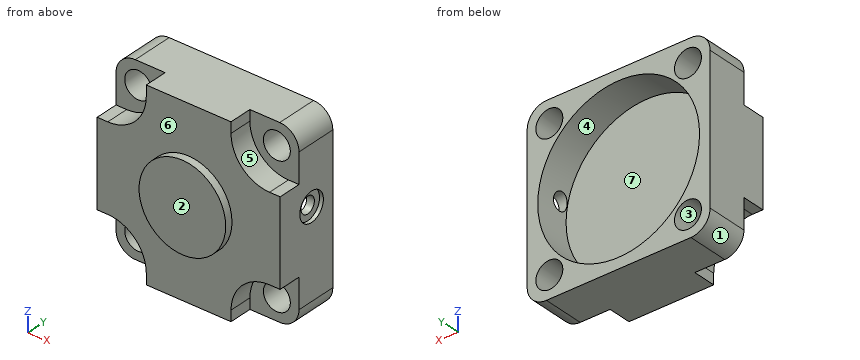
from build123d import *

# Parameters (mm, degrees)
F0_R      = 7
F1_DEPTH  = 16.75
F2_R      = 7
F3_DEPTH  = 12
F4_R      = 22.5
F5_DEPTH  = 4
F6_R      = 42
F8_DEPTH  = 18
F7_R      = 7.5
F7_R_2    = 4.25
F9_DEPTH  = 2
F10_DEPTH = 8


with BuildPart() as f1:
    # F0 (on Front) → F1 (new body, symmetric)
    with BuildSketch(Plane.XZ):
        with BuildLine():
            Line((-37.5, -47.5), (37.5, -47.5))
            ThreePointArc((37.5, -47.5), (44.5710678119, -44.5710678119), (47.5, -37.5))
            Line((47.5, -37.5), (47.5, 37.5))
            ThreePointArc((47.5, 37.5), (44.5710678119, 44.5710678119), (37.5, 47.5))
            Line((37.5, 47.5), (-37.5, 47.5))
            ThreePointArc((-37.5, 47.5), (-44.5710678119, 44.5710678119), (-47.5, 37.5))
            Line((-47.5, 37.5), (-47.5, -37.5))
            ThreePointArc((-47.5, -37.5), (-44.5710678119, -44.5710678119), (-37.5, -47.5))
        make_face()
        with Locations((-36, -36)):
            Circle(F0_R, mode=Mode.SUBTRACT)
        with Locations((36, -36)):
            Circle(F0_R, mode=Mode.SUBTRACT)
        with Locations((-36, 36)):
            Circle(F0_R, mode=Mode.SUBTRACT)
        with Locations((36, 36)):
            Circle(F0_R, mode=Mode.SUBTRACT)
    extrude(amount=F1_DEPTH, both=True)

    # F2 (on face) → F3 (cut)
    with BuildSketch(Plane.XZ.offset(16.75)):
        with BuildLine():
            Line((22, -42), (22, -47.5))
            Line((22, -47.5), (37.5, -47.5))
            ThreePointArc((37.5, -47.5), (44.5710678119, -44.5710678119), (47.5, -37.5))
            Line((47.5, -37.5), (47.5, -22))
            Line((47.5, -22), (42, -22))
            ThreePointArc((42, -22), (27.8578643763, -27.8578643763), (22, -42))
        make_face()
        with Locations((36, -36)):
            Circle(F2_R, mode=Mode.SUBTRACT)
        with BuildLine():
            Line((37.5, 47.5), (22, 47.5))
            Line((22, 47.5), (22, 42))
            ThreePointArc((22, 42), (27.8578643763, 27.8578643763), (42, 22))
            Line((42, 22), (47.5, 22))
            Line((47.5, 22), (47.5, 37.5))
            ThreePointArc((47.5, 37.5), (44.5710678119, 44.5710678119), (37.5, 47.5))
        make_face()
        with Locations((36, 36)):
            Circle(F2_R, mode=Mode.SUBTRACT)
        with BuildLine():
            Line((-47.5, 37.5), (-47.5, 22))
            Line((-47.5, 22), (-42, 22))
            ThreePointArc((-42, 22), (-27.8578643763, 27.8578643763), (-22, 42))
            Line((-22, 42), (-22, 47.5))
            Line((-22, 47.5), (-37.5, 47.5))
            ThreePointArc((-37.5, 47.5), (-44.5710678119, 44.5710678119), (-47.5, 37.5))
        make_face()
        with Locations((-36, 36)):
            Circle(F2_R, mode=Mode.SUBTRACT)
        with BuildLine():
            Line((-42, -22), (-47.5, -22))
            Line((-47.5, -22), (-47.5, -37.5))
            ThreePointArc((-47.5, -37.5), (-44.5710678119, -44.5710678119), (-37.5, -47.5))
            Line((-37.5, -47.5), (-22, -47.5))
            Line((-22, -47.5), (-22, -42))
            ThreePointArc((-22, -42), (-27.8578643763, -27.8578643763), (-42, -22))
        make_face()
        with Locations((-36, -36)):
            Circle(F2_R, mode=Mode.SUBTRACT)
    extrude(amount=-F3_DEPTH, mode=Mode.SUBTRACT)

    # F4 (on face) → F5 (join)
    with BuildSketch(Plane.XZ.offset(16.75)):
        Circle(F4_R)
    extrude(amount=F5_DEPTH)

    # F6 (on face) → F8 (cut)
    with BuildSketch(Plane(origin=(0, 16.75, 0), x_dir=(-1, 0, 0), z_dir=(0, 1, 0))):
        Circle(F6_R)
    extrude(amount=-F8_DEPTH, mode=Mode.SUBTRACT)

    # F7 (on face) → F9 (cut)
    with BuildSketch(Plane.YZ.offset(47.5)):
        with Locations((3.25, 7.547759451)):
            Circle(F7_R)
        with Locations((3.25, 7.547759451)):
            Circle(F7_R_2, mode=Mode.SUBTRACT)
    extrude(amount=-F9_DEPTH, mode=Mode.SUBTRACT)

    # F10 (cut): a face of the model
    f10_faces = [f1.faces().sort_by_distance(p)[0] for p in [
        (47.5, 3.25, 7.547759451),
    ]]
    extrude(f10_faces, amount=-F10_DEPTH, mode=Mode.SUBTRACT)


solid = f1.part
Build history of the part. All positions in model axes, mm. Face numbers are marked on the shaded views. A direction names the side the tool comes from. Coordinates: 2 decimals unless noted, no trailing zeros. Order: outer loops, then holes, each group sorted by start corner. A loop starts at its lowest first (then second) coordinate and runs counter-clockwise, first axis right, second up. Notation, with made-up numbers: (8, 76.25) - (35, 76.25) arc R14 cw to (35, 99.25) - close; hole circle Ø6 at (57.5, 67). An arc over 180 degrees is marked (long way). Write item = value, one per line. Start each with the question number.
1) Two-plate mould, pull along X, no slides. Class the marked faces 1, 2, 3 and 4: pulls with the +X half, pulls with the -X half, needs draft (parallel to the pull), parting line crosses it, or undercut.
2) Saw through at C-C on x = 36. Write the cut outline in (y, z).
3) Saw through at B-B on z = 40.5. Write the cut outline in (x, y).
4) Flat gauge pins, fed straight in: pin 1 Ø4.5 at (y, z) = (-10.5, -46) entering from -X; pin 2 Ø6 at (x, y) = (-44.5, -10.5) entering from +Z; pin 3 Ø6 at (y, z) = (-10.5, 44.5) entering from +X; pin 4 Ø22.5 at (x, z) = (-36, 36) entering from +Y. Where does each tip first touch, or does it go through?
5) Saw through at A-A on y = 14. Write the cut outline in (x, z).
6) Saw through at D-D on x = 0. Write the cut outline in (y, z), then the cut area to 3 significant figures.
7) 3-axis set-ups, long thin cutter, end or side, ignore diameter. For the marked faces 5, 6 and 7: which of +Z, -Z, +X, -X, +Y, -Y reach the whole face in a straight line?
8) Wall check: line 1 along Z through (x, y) = (36, 7.5); line 2 along X through (y, z) = (6.5, -31); line 3 along X through (y, z) = (7, 30). Give the ranges that are in metal, low to high. Write a range as from..to.
From the geometry:
q1.face_1 = pulls with the -X half
q1.face_2 = needs draft
q1.face_3 = undercut
q1.face_4 = undercut
q2.outline = (-16.75, -22.92) - (-4.75, -22.92) - (-4.75, -29) - (16.75, -29) - (16.75, -21.63) - (-1.25, -21.63) - (-1.25, 21.63) - (16.75, 21.63) - (16.75, 29) - (-4.75, 29) - (-4.75, 22.92) - (-16.75, 22.92) - close; (-4.75, -47.5) - (16.75, -47.5) - (16.75, -43) - (-4.75, -43) - close; (-4.75, 43) - (16.75, 43) - (16.75, 47.5) - (-4.75, 47.5) - close
q3.outline = (-47.04, -4.75) - (-41.36, -4.75) - (-41.36, 16.75) - (-47.04, 16.75) - close; (-30.64, -4.75) - (-22.06, -4.75) - (-22.06, -16.75) - (22.06, -16.75) - (22.06, -4.75) - (30.64, -4.75) - (30.64, 16.75) - (11.12, 16.75) - (11.12, -1.25) - (-11.12, -1.25) - (-11.12, 16.75) - (-30.64, 16.75) - close; (41.36, -4.75) - (47.04, -4.75) - (47.04, 16.75) - (41.36, 16.75) - close
q4.pin_1 = -22
q4.pin_2 = 22.01
q4.pin_3 = 22.01
q4.pin_4 = 16.75
q5.outline = (-47.5, -37.5) arc R10 ccw to (-37.5, -47.5) - (37.5, -47.5) arc R10 ccw to (47.5, -37.5) - (47.5, 37.5) arc R10 ccw to (37.5, 47.5) - (-37.5, 47.5) arc R10 ccw to (-47.5, 37.5) - close; hole circle Ø14 at (-36, -36); hole circle Ø14 at (-36, 36); hole circle Ø84 at (0, 0); hole circle Ø14 at (36, -36); hole circle Ø14 at (36, 36)
q6.outline = (-20.75, -22.5) - (-16.75, -22.5) - (-16.75, -47.5) - (16.75, -47.5) - (16.75, -42) - (-1.25, -42) - (-1.25, 42) - (16.75, 42) - (16.75, 47.5) - (-16.75, 47.5) - (-16.75, 22.5) - (-20.75, 22.5) - close
q6.area = 1,850 mm^2
q7.face_5 = +Z, +X, -Y
q7.face_6 = -Y
q7.face_7 = +Y
q8.line_1 = -47.5..-43, -29..-21.63, 21.63..29, 43..47.5
q8.line_2 = -47.5..-40.9, -31.1..-28.34, 28.34..31.1, 40.9..47.5
q8.line_3 = -47.5..-39.61, -32.39..-29.39, 29.39..32.39, 39.61..47.5
